Autodesk Inventor part; units mm, degrees
ref_plane "Work Plane1" through (0, -15.875, 0) normal (0, 1, 0) x (-1, 0, 0)
ref_plane "Work Plane2" through (15.875, 0, 0) normal (1, 0, 0) x (0, 1, 0)
ref_plane "XY Plane" through (0, 0, 0) normal (0, 0, 1) x (1, 0, 0)
sketch "Sketch1" plane through (0, 0, 0) normal (0, 0, 1) x (1, 0, 0)
  circle A0 centre (0, 0) radius 15.875
  circle A1 centre (0, 0) radius 14.2875
  dimension "d0" = 31.75
  dimension "d1" = 28.575
extrude "Extrusion1" add sketch "Sketch1" along normal blind 254
ref_plane "Work Plane1" through (0, -15.875, 0) normal (0, 1, 0) x (-1, 0, 0)
sketch "Sketch2" plane through (0, -15.875, 0) normal (0, 1, 0) x (-1, 0, 0)
  line L0 (15.875, 254) -> (-15.875, 254)
  line L1 (-15.875, 0) -> (15.875, 0)
  line L2 (18.6459, 127) -> (-13.1041, 127) construction
  line L3 (15.875, 0) -> (15.875, 254) construction
  line L4 (-15.875, 0) -> (-15.875, 254) construction
  circle A0 centre (0, 5.5563) radius 2.413
  circle A1 centre (0, 248.4437) radius 2.413
  point P0 (0, 0)
  dimension "d4" = 127
  dimension "d5" = 4.826
  dimension "d6" = 5.5563
  dimension "d7" = 15.875
extrude "Extrusion2" cut sketch "Sketch2" along normal blind 50.8
ref_plane "Work Plane2" through (15.875, 0, 0) normal (1, 0, 0) x (0, 1, 0)
sketch "Sketch3" plane through (15.875, 0, 0) normal (1, 0, 0) x (0, 1, 0)
  line L0 (-15.875, 0) -> (15.875, 0)
  line L1 (15.875, 0) -> (15.875, 254)
  line L2 (-15.875, 0) -> (-15.875, 254)
  line L3 (15.875, 254) -> (-15.875, 254)
  line L4 (15.875, 127) -> (-15.875, 127) construction
  circle A0 centre (0, 5.5563) radius 2.413
  circle A1 centre (0, 248.4437) radius 2.413
  point P0 (0, 0)
  dimension "d10" = 127
  dimension "d11" = 4.826
  dimension "d12" = 5.5563
  dimension "d13" = 15.875
extrude "Extrusion3" cut sketch "Sketch3" against normal blind 50.8 contours A0 | A1
equation "\"d4\" = 0.5 * d2"
equation "\"d10\" = 0.5 * d2"
properties part number "Polycarbonate Roller 1.25 OD 1.125 ID (8585K63)" material "Polycarbonate, Clear"
CAD build for the part. Positions are in the model's coordinates, mm. Coordinates: 2 decimals unless noted, no trailing zeros. Order: outer loops, then holes, each group sorted by start corner. A loop starts at its lowest first (then second) coordinate and runs counter-clockwise, first axis right, second up. Notation, with made-up numbers: M -40,6 L 16,6 A24 ccw 16,45 Z; hole C 18,47 d2. An arc over 180 degrees is marked long. Write each question's results on one line, items separated by ' | '. Start each with the question number.
Q1. Cut at C-C (y = -11.5). List the corners of the cut face in (x, z).
Q2. Pull direction Z, two halves, no side cores. Call faces 1 (the flat face through (-11.83, 8.31, 0)), 2 (the flat face through (-11.83, 8.31, 254)), 3 (the cylindrical face through (-1.3, 14.97, 246.41)): +Z half, -Z half, draft (parallel to the pull), parting line (faces both ways), or undercut.
Q3. Drill centre lines: probe 1 along Z at (x, y) = (15, 0); probe 2 along X at (y, z) = (0, 55) (1 decimal); probe 3 along Y at (x, z) = (-1, 170). Where is each one in solid material? Low to high. Write a range as from..to.
Q4. Cut at A-A (y = 0). List the corners of the cut face in (x, z) (1 decimal).
Q5. Cut at D-D (x = -12). List the corners of the cut face in (y, z), then the cut area to 3 significant figures.
Q6. Flat gauge pins, fed straight in: P1, Ø1.5, axis at x = -4, z = 155, coming from the -Y side; P2, Ø6, axis at y = 11.5, z = 153.5, coming from the +X side; P3, Ø8, axis at y = -7, z = 123, coming from the +X side. Where does each tip first touch, or does it go through?
Found:
1) outline: M -10.94,0 L -8.48,0 L -8.48,254 L -10.94,254 Z; M 8.48,0 L 10.94,0 L 10.94,254 L 8.48,254 Z
2) face 1: -Z half | face 2: +Z half | face 3: undercut
3) probe 1: 0..3.14, 7.97..246.03, 250.86..254 | probe 2: -15.9..-14.3, 14.3..15.9 | probe 3: -15.84..-14.25, 14.25..15.84
4) outline: M -15.9,0 L -14.3,0 L -14.3,3.1 L -15.9,3.1 Z; M -15.9,8 L -14.3,8 L -14.3,246 L -15.9,246 Z; M -15.9,250.9 L -14.3,250.9 L -14.3,254 L -15.9,254 Z; M 14.3,0 L 15.9,0 L 15.9,3.1 L 14.3,3.1 Z; M 14.3,8 L 15.9,8 L 15.9,246 L 14.3,246 Z; M 14.3,250.9 L 15.9,250.9 L 15.9,254 L 14.3,254 Z
5) outline: M -10.39,0 L -7.75,0 L -7.75,254 L -10.39,254 Z; M 7.75,0 L 10.39,0 L 10.39,254 L 7.75,254 Z | area: 1,340 mm²
6) P1: y = -15.54 | P2: x = 13.41 | P3: x = 15.59
